Verification items for the finished model (mm, model axes). Face numbers are marked on the shaded views. A direction names the side the tool comes from. Round coordinates to 2 decimals unless told otherwise and drop trailing zeros. Loops run counter-clockwise (first coordinate to the right, second up) from the corner with the lowest first, then second, coordinate; pieces in that order, holes last. Notation, with made-up numbers: M -18,9.25 L -12,9.25 A22 cw -12,47.25 Z; hole C -34.5,22.5 d2. An arc over 180 degrees is marked long. One line per item, written item: value.
from build123d import *

# Parameters (mm, degrees)
F1_START     = -88.9
F0_R         = 18.415
F0_R_2       = 12.7
F1_DEPTH     = 12.7
F2_START     = -83.82
F2_DEPTH     = 2.54
F3_START     = -78.74
F3_DEPTH     = 2.54
F4_START     = -73.66
F4_DEPTH     = 2.54
F5_START     = -68.58
F5_DEPTH     = 2.54
F6_START     = -63.5
F6_DEPTH     = 2.54
F7_START     = -58.42
F7_DEPTH     = 2.54
F8_DEPTH     = 55.88
F9_R         = 15.24
F9_R_2       = 12.7
F10_DEPTH    = 101.6
F11_S5_R     = 15.24
F11_T6_DEPTH = 28
F12_S5_R     = 15.24
F12_T6_DEPTH = 53
F13_START    = -88.9
F13_DEPTH    = 2.54
F14_DEPTH    = 50.8


# Not quite as in the source:
# - a fillet or chamfer that OpenCascade refuses, or shapes differently, is made with other operations: its cross-section is extruded or revolved along the edge and cut away or added


with BuildPart() as f1:
    # F0 (on Front) → F1 (new body)
    with BuildSketch(Plane.XZ.offset(F1_START)):
        Circle(F0_R)
        Circle(F0_R_2, mode=Mode.SUBTRACT)
    extrude(amount=-F1_DEPTH)



with BuildPart() as f2:
    # F0 (on Front) → F2 (new body)
    with BuildSketch(Plane.XZ.offset(F2_START)):
        Circle(F0_R)
        Circle(F0_R_2, mode=Mode.SUBTRACT)
    extrude(amount=-F2_DEPTH)


with BuildPart() as f3:
    # F0 (on Front) → F3 (new body)
    with BuildSketch(Plane.XZ.offset(F3_START)):
        Circle(F0_R)
        Circle(F0_R_2, mode=Mode.SUBTRACT)
    extrude(amount=-F3_DEPTH)


with BuildPart() as f4:
    # F0 (on Front) → F4 (new body)
    with BuildSketch(Plane.XZ.offset(F4_START)):
        Circle(F0_R)
        Circle(F0_R_2, mode=Mode.SUBTRACT)
    extrude(amount=-F4_DEPTH)


with BuildPart() as f5:
    # F0 (on Front) → F5 (new body)
    with BuildSketch(Plane.XZ.offset(F5_START)):
        Circle(F0_R)
        Circle(F0_R_2, mode=Mode.SUBTRACT)
    extrude(amount=-F5_DEPTH)


with BuildPart() as f6:
    # F0 (on Front) → F6 (new body)
    with BuildSketch(Plane.XZ.offset(F6_START)):
        Circle(F0_R)
        Circle(F0_R_2, mode=Mode.SUBTRACT)
    extrude(amount=-F6_DEPTH)


with BuildPart() as f7:
    # F0 (on Front) → F7 (new body)
    with BuildSketch(Plane.XZ.offset(F7_START)):
        Circle(F0_R)
        Circle(F0_R_2, mode=Mode.SUBTRACT)
    extrude(amount=-F7_DEPTH)


with BuildPart() as f8:
    # F0 (on Front) → F8 (new body)
    with BuildSketch(Plane.XZ):
        Circle(F0_R)
        Circle(F0_R_2, mode=Mode.SUBTRACT)
    extrude(amount=-F8_DEPTH)


with BuildPart() as f1_1:
    add(f1.part)

    add(f2.part)  # F10 merges F2

    add(f3.part)  # F10 merges F3

    add(f4.part)  # F10 merges F4

    add(f5.part)  # F10 merges F5

    add(f6.part)  # F10 merges F6

    add(f7.part)  # F10 merges F7

    add(f8.part)  # F10 merges F8
    # F9 (on Front) → F10 (join)
    with BuildSketch(Plane.XZ):
        Circle(F9_R)
        Circle(F9_R_2, mode=Mode.SUBTRACT)
    extrude(amount=-F10_DEPTH)

    # F11: chamfer of 2.54 x 3.81 on 1 edges, made by hand


with BuildPart() as f11_tool2:
    # F11_s3 → F11_t4 (revolve)
    with BuildSketch(Plane.XY):
        Polygon((18.415, 53.34), (14.605, 55.88), (18.415, 55.88), align=None)
    revolve(axis=Axis((0, 55.88, 0), (0, -1, 0)))

    # F11_s5 → F11_t6 (cut, symmetric)
    with BuildSketch(Plane.XZ.offset(-54.6)):
        Circle(F11_S5_R)
    extrude(amount=F11_T6_DEPTH, both=True, mode=Mode.SUBTRACT)


with BuildPart() as f1_2:
    add(f1_1.part)

    # F11_t1: cut F11_tool2
    add(f11_tool2.part, mode=Mode.SUBTRACT)

    # F12: chamfer of 12.7 x 7.62 on 1 edges, made by hand


with BuildPart() as f12_tool2:
    # F12_s3 → F12_t4 (revolve)
    with BuildSketch(Plane.XY):
        with BuildLine():
            Line((5.2793935937, 88.6386361562), (18.8506064063, 96.7813638438))
            Line((18.8506064063, 96.7813638438), (19.1046064063, 96.7813638438))
            ThreePointArc((19.1046064063, 96.7813638438), (18.669, 92.8406819219), (18.669, 88.9))
            Line((18.669, 88.9), (18.415, 88.646))
            ThreePointArc((18.415, 88.646), (11.8471967969, 88.646), (5.2793935937, 88.3846361562))
            Line((5.2793935937, 88.3846361562), (5.2793935937, 88.6386361562))
        make_face()
    revolve(axis=Axis((0, 88.9, 0), (0, -1, 0)))

    # F12_s5 → F12_t6 (cut, symmetric)
    with BuildSketch(Plane.XZ.offset(-90.9)):
        Circle(F12_S5_R)
    extrude(amount=F12_T6_DEPTH, both=True, mode=Mode.SUBTRACT)


with BuildPart() as f1_3:
    add(f1_2.part)

    # F12_t1: cut F12_tool2
    add(f12_tool2.part, mode=Mode.SUBTRACT)

    # F0 (on Front) → F13 (join)
    with BuildSketch(Plane.XZ.offset(F13_START)):
        Circle(F0_R)
        Circle(F0_R_2, mode=Mode.SUBTRACT)
    extrude(amount=-F13_DEPTH)

    # F0 (on Front) → F14 (cut)
    with BuildSketch(Plane.XZ):
        Circle(F0_R)
        Circle(F0_R_2, mode=Mode.SUBTRACT)
    extrude(amount=-F14_DEPTH, mode=Mode.SUBTRACT)


solid = f1_3.part
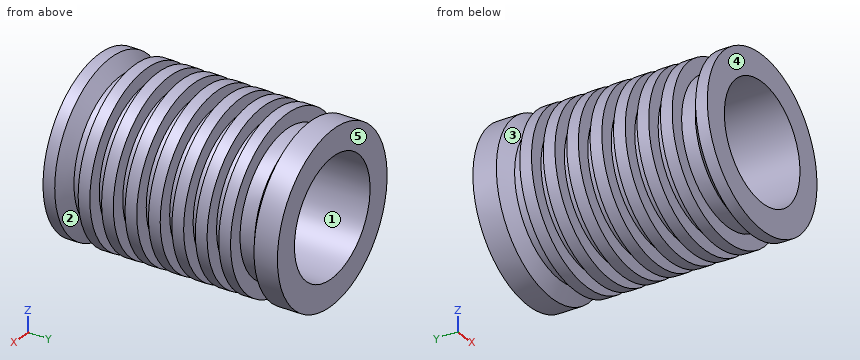
(1) Sectioned sample at A-A on y = 85.5. Enter the section's corners in (x, z) (3 decimals).
Completed:
outline: C 0,0 d36.83; hole C 0,0 d25.4
(2) Tool access check on the marked faces 1 and 2. Record the directions out of +Z, -Z, +X, -X, +Y, -Y that give a thin tool (end or side, any length) a straight path to the whole face; none if there is none.
Completed:
face 1: +Y, -Y
face 2: none
(3) Mould release check, pull along Y, two halves, no side actions. Record for the marked faces 3, 4 and 5: +Y half, -Y half, draft (parallel to the pull), parting line (faces both ways), or undercut.
Completed:
face 3: undercut
face 4: -Y half
face 5: +Y half
(4) Sectioned sample at B-B on x = -16. Count the separate pieces of the cut face and the enclosed holes in it, and give its area (3 significant figures).
Completed:
separate pieces: 9
enclosed holes: 0
area: 500 mm^2
(5) Depth check by flat-ended pin: pin 1 Ø6 at (y, z) = (81, 6) entering from -X; pin 2 Ø3 at (x, y) = (14.5, 72.5) entering from -Z; pin 3 Ø11 at (x, z) = (-7, 0.5) entering from -Y (3 decimals); pin 4 Ø1 at (y, z) = (60.5, -6) entering from -X. Enter the tip coordinate at first touch or a pass-through.
Completed:
pin 1: stops at x = -18.17
pin 2: stops at z = -12.47
pin 3: passes through
pin 4: stops at x = -17.57
(6) Thickness scan on L1, parallel to Z at x = 0, y = 73; L2, parallel to Z at x = 0, y = 81 (3 decimals); L3, parallel to X at y = 79.5, z = -0.5. Record the ranges inside material, lowest first. Write a range as from..to.
Completed:
L1: z = -15.24..-12.7, 12.7..15.24
L2: z = -18.415..-12.7, 12.7..18.415
L3: x = -18.41..-12.69, 12.69..18.41
(7) Sectioned sample at C-C on y = 93. Enter the section's corners in (x, z).
Completed:
outline: C 0,0 d30.48; hole C 0,0 d25.4
